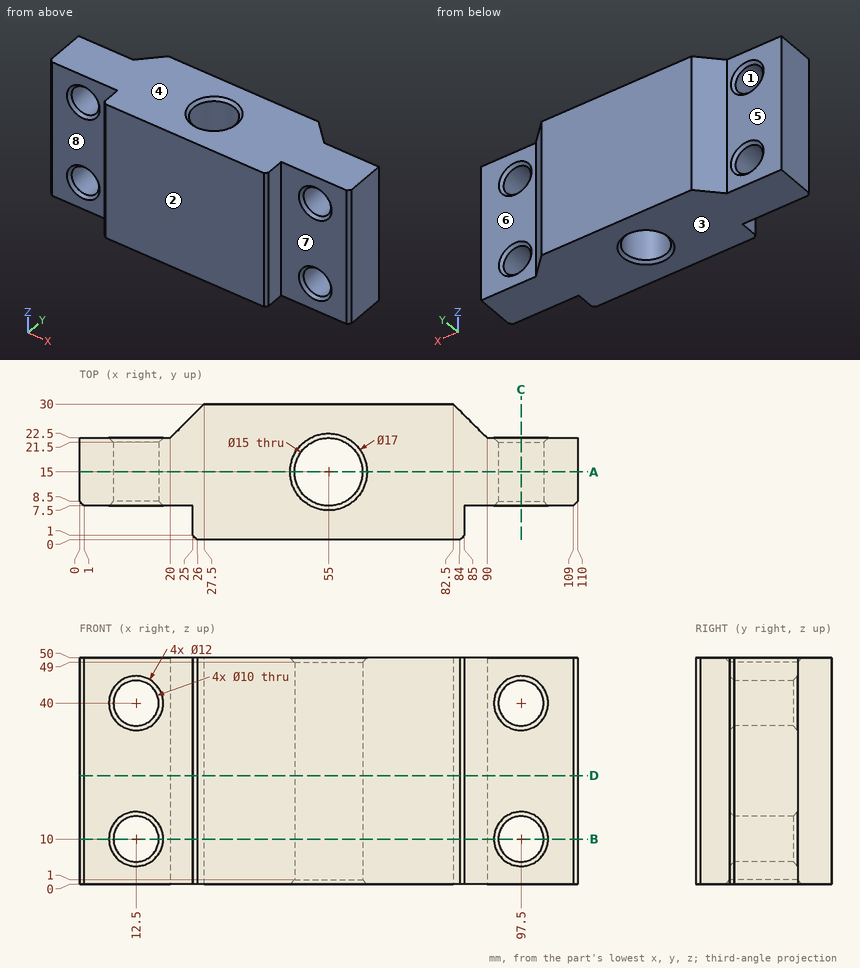
The figure shows three views and two pictorial views of one solid part (mm, origin at its lowest corner). Answer the questions. A direction names the side the tool comes from. Coordinates: 2 decimals unless noted, no trailing zeros. Loops run counter-clockwise (first coordinate to the right, second up) from the corner with the lowest first, then second, coordinate; pieces in that order, holes last. Notation, with made-up numbers: (-29, -22.5) - (22, -22.5) arc R22 ccw to (22, 3.5) - close; hole circle Ø5 at (26.5, 77). An arc over 180 degrees is marked (long way). Use a Markdown table: item, result. Add a question column.
1) The part is cut by section A-A, the plane y = 15. Give the vertices of the cut face in (x, z), and give its area (3 significant figures).
2) The part is cut by section C-C, the plane x = 97.5. Give the vertices of the cut face in (y, z), and give its area (3 significant figures).
3) The part is cut by section D-D, the plane z = 24. Give the vertices of the cut face in (x, y).
4) Find the intervals of material crossed by line 1 (Z direction, x = 97.5, y = 15.25); line 2 (Z direction, x = 8, y = 21.5); line 3 (X direction, y = 14.5, z = 4.5), in increasing order.
5) The part is cut by section B-B, the plane z = 10. State how many separate pieces and enclosed holes the cut face has, and give its area (3 significant figures).
6) Given pin 1 (9 mm diameter, centred on x = 12.5, z = 40, fed in from +Y); pin 2 (12 mm diameter, centred on x = 99.5, z = 25, fed in from -Y); pin 3 (6 mm diameter, centred on x = 97.5, z = 12.5, fed in from +Y); pin 4 (3 mm diameter, centred on y = 26.5, z = 7.5, fed in from +X), each flat-ended and moving along its own axis, determine where each tip first touches the part or whether it passes through.
7) The mould has two halves that part along Z. Classify the marked faces 1, 2, 3 and 4: released by +Z, released by -Z, zero draft, split by the parting line, or undercut.
8) For the marked faces 5, 6, 7 and 8, determine the directions among +Z, -Z, +X, -X, +Y, -Y from which every point of the face is accessible in a straight line to the end or side of a thin tool.
Here are the results:
| question | item | result |
|---|---|---|
| 1 | outline | (0, 0) - (46.5, 0) - (47.5, 1) - (47.5, 49) - (46.5, 50) - (0, 50) - close; (62.5, 1) - (63.5, 0) - (110, 0) - (110, 50) - (63.5, 50) - (62.5, 49) - close; hole circle Ø10 at (12.5, 10); hole circle Ø10 at (12.5, 40); hole circle Ø10 at (97.5, 10); hole circle Ø10 at (97.5, 40) |
| 1 | area | 4,430 mm^2 |
| 2 | outline | (7.5, 0) - (22.5, 0) - (22.5, 4) - (21.5, 5) - (8.5, 5) - (7.5, 4) - close; (7.5, 16) - (8.5, 15) - (21.5, 15) - (22.5, 16) - (22.5, 34) - (21.5, 35) - (8.5, 35) - (7.5, 34) - close; (7.5, 46) - (8.5, 45) - (21.5, 45) - (22.5, 46) - (22.5, 50) - (7.5, 50) - close |
| 2 | area | 446 mm^2 |
| 3 | outline | (0, 8.5) - (1, 7.5) - (25, 7.5) - (25, 1) - (26, 0) - (84, 0) - (85, 1) - (85, 7.5) - (109, 7.5) - (110, 8.5) - (110, 22.5) - (90, 22.5) - (82.5, 30) - (27.5, 30) - (20, 22.5) - (0, 22.5) - close; hole circle Ø15 at (55, 15) |
| 4 | line 1 | z = 0 to 5, 15 to 35, 45 to 50 |
| 4 | line 2 | z = 0 to 7.82, 12.18 to 37.82, 42.18 to 50 |
| 4 | line 3 | x = 0 to 47.52, 62.48 to 110 |
| 5 | separate pieces | 3 |
| 5 | enclosed holes | 1 |
| 5 | area | 2,090 mm^2 |
| 6 | pin 1 | passes through |
| 6 | pin 2 | stops at y = 7.5 |
| 6 | pin 3 | stops at y = 22 |
| 6 | pin 4 | stops at x = 87.5 |
| 7 | face 1 | undercut |
| 7 | face 2 | zero draft |
| 7 | face 3 | released by -Z |
| 7 | face 4 | released by +Z |
| 8 | face 5 | +Z, -Z, -X, +Y |
| 8 | face 6 | +Z, -Z, +X, +Y |
| 8 | face 7 | +Z, -Z, +X, -Y |
| 8 | face 8 | +Z, -Z, -X, -Y |
